from build123d import *

# Parameters (mm, degrees)
CROQUIS1_R              = 16
CROQUIS1_R_2            = 6
CROQUIS1_R_3            = 1.5
SALIENTE_EXTRUIR1_DEPTH = 2.2
CROQUIS1_3_R            = 6
CROQUIS1_3_R_2          = 2
SALIENTE_EXTRUIR2_DEPTH = 3.2
CROQUIS1_4_R            = 2
SALIENTE_EXTRUIR3_DEPTH = 11.4
CROQUIS5_W              = 8
CROQUIS5_H              = 20.560227787
SALIENTE_EXTRUIR4_DEPTH = 0.3


with BuildPart() as part:
    # Croquis1 → Saliente-Extruir1 (new body)
    with BuildSketch(Plane(origin=(0, 0, 0), x_dir=(1, 0, 0), z_dir=(0, 1, 0))):
        with Locations(Location((0, 0, 0), (0, 0, 270))):
            Circle(CROQUIS1_R)
        with Locations(Location((0, 0, 0), (0, 0, 270))):
            Circle(CROQUIS1_R_2, mode=Mode.SUBTRACT)
        with Locations(Location((0, 12, 0), (0, 0, 270))):
            Circle(CROQUIS1_R_3, mode=Mode.SUBTRACT)
        with Locations(Location((10.392304845, -6, 0), (0, 0, 270))):
            Circle(CROQUIS1_R_3, mode=Mode.SUBTRACT)
        with Locations(Location((-10.392304845, -6, 0), (0, 0, 270))):
            Circle(CROQUIS1_R_3, mode=Mode.SUBTRACT)
    extrude(amount=SALIENTE_EXTRUIR1_DEPTH)



with BuildPart() as body_2:
    # Croquis1_3 → Saliente-Extruir2 (new body)
    with BuildSketch(Plane(origin=(0, 0, 0), x_dir=(1, 0, 0), z_dir=(0, 1, 0))):
        with Locations(Location((0, 0, 0), (0, 0, 270))):
            Circle(CROQUIS1_3_R)
        with Locations(Location((0, 0, 0), (0, 0, 270))):
            Circle(CROQUIS1_3_R_2, mode=Mode.SUBTRACT)
    extrude(amount=SALIENTE_EXTRUIR2_DEPTH)


with BuildPart() as part_1:
    add(part.part)

    add(body_2.part)  # Saliente-Extruir3 merges body 2
    # Croquis1_4 → Saliente-Extruir3 (add)
    with BuildSketch(Plane(origin=(0, 0, 0), x_dir=(1, 0, 0), z_dir=(0, 1, 0))):
        with Locations(Location((0, 0, 0), (0, 0, 270))):
            Circle(CROQUIS1_4_R)
    extrude(amount=SALIENTE_EXTRUIR3_DEPTH)

    # Croquis4 → Revoluci_n1 (revolve)
    with BuildSketch(Plane(origin=(0, 0, 0), x_dir=(0, 0, -1), z_dir=(1, 0, 0)), mode=Mode.PRIVATE) as revoluci_n1_sk:
        Polygon((15.909149683, -0.847381969), (15.909149683, -0.322612836), (16, -0.322612836), (16, 0), (0, 0), (0, -16.5), (1, -16.5), (1.1, -16.5), (16, -16.5), (16, -0.847381969), align=None)
    revolve(revoluci_n1_sk.sketch.rotate(Axis((0, 0, 0), (0, -1, 0)), 180), axis=Axis((0, 0, 0), (0, -1, 0)))

    # Croquis5 → Saliente-Extruir4 (add)
    with BuildSketch(Plane(origin=(0, -0.322612836, 0), x_dir=(-1, 0, 0), z_dir=(0, -1, 0))):
        with Locations((0, -19.361082391)):
            Rectangle(CROQUIS5_W, CROQUIS5_H)
    extrude(amount=-SALIENTE_EXTRUIR4_DEPTH)


solid = part_1.part
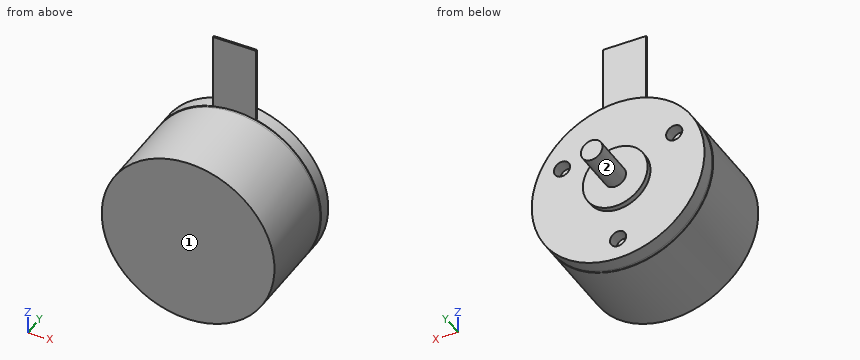
Geometry: final body of the model. Coordinates: model frame, mm. Face numbers are marked on the shaded views. A direction names the side the tool comes from. Round coordinates to 2 decimals unless told otherwise and drop trailing zeros. Write each loop counter-clockwise with the first axis right and the second up, starting at its lowest first coordinate (ties: lowest second). Pieces come first, ordered by that corner, then holes. Notation, with made-up numbers: M -13.75,66 L 31.25,66 A24 cw 31.25,95 Z; hole C 56,72.5 d7. An arc over 180 degrees is marked long. Write item = value, one per line.
Item 1: Material intervals for line 1 along X through (y, z) = (1.2, 6); line 2 along X through (y, z) = (0.5, -12); line 3 along Y through (x, z) = (9, -0.5), sorted ascending. Write a range as [from, to].
Findings:
line_1 = [-14.83, -11.89], [-8.89, 8.89], [11.89, 14.83]
line_2 = [-10.58, -1.5], [1.5, 10.58]
line_3 = [-16.5, 2.2]
Item 2: Section query C-C on y = -14. Return loops of the section in (x, z), then the cut area to 3 significant figures.
Findings:
outline = C 0,0 d32
area = 804 mm^2
Item 3: Pin query (flat end, axial travel): P1, Ø3.5, axis at x = 11, z = 6, coming from the +Y side; P2, Ø2.5, axis at x = 1.5, z = 26, coming from the +Y side; P3, Ø5, axis at y = -4, z = 14, coming from the -X side. Return the tip coordinate at first contact, or that it passes through.
Findings:
P1 = 2.2
P2 = -0.02
P3 = -11.12
Item 4: Section query D-D on z = 3. Return loops of the section in (x, y), then the cut area to 3 significant figures.
Findings:
outline = M -15.72,-16.5 L 15.72,-16.5 L 15.72,-0.85 L 15.62,-0.85 L 15.62,-0.32 L 15.72,-0.32 L 15.72,2.2 L 5.2,2.2 L 5.2,3.2 L -5.2,3.2 L -5.2,2.2 L -15.72,2.2 L -15.72,-0.32 L -15.62,-0.32 L -15.62,-0.85 L -15.72,-0.85 Z
area = 598 mm^2
Item 5: Section query B-B on z = -12. Return loops of the section in (x, y), then the cut area to 3 significant figures.
Findings:
outline = M -10.58,-16.5 L 10.58,-16.5 L 10.58,-0.85 L 10.45,-0.85 L 10.45,-0.32 L 10.58,-0.32 L 10.58,2.2 L 1.5,2.2 L 1.5,0 L -1.5,0 L -1.5,2.2 L -10.58,2.2 L -10.58,-0.32 L -10.45,-0.32 L -10.45,-0.85 L -10.58,-0.85 Z
area = 389 mm^2
Item 6: Access query for the marked faces 1 and 2. Directions: +Z, -Z, +X, -X, +Y, -Y. A direction counts if a zero-diameter tool reaches every point of the face in a straight line with its end or side. Return the directions, or none.
Findings:
face_1 = +Z, -Z, +X, -X, -Y
face_2 = +Y
Item 7: Section query A-A on x = 0. Return loops of the section in (y, z).
Findings:
outline = M -16.5,-16 L -0.85,-16 L -0.85,-15.91 L -0.32,-15.91 L -0.32,-16 L 2.2,-16 L 2.2,-13.5 L 0,-13.5 L 0,-10.5 L 2.2,-10.5 L 2.2,-6 L 3.2,-6 L 3.2,-2 L 11.4,-2 L 11.4,2 L 3.2,2 L 3.2,6 L 2.2,6 L 2.2,16 L -0.02,16 L -0.02,29.64 L -0.32,29.64 L -0.32,15.91 L -0.85,15.91 L -0.85,16 L -16.5,16 Z
